Verification items for the finished model (mm, model axes). A direction names the side the tool comes from. Give positions to 0.01 mm unless a question says otherwise; leave off trailing zeros. Write each loop counter-clockwise with the first axis right and the second up, starting at its lowest first coordinate (ties: lowest second). Pieces come first, ordered by that corner, then holes. Notation, with made-up numbers: M -27.75,71.5 L 12.25,71.5 A25 cw 12.25,92.5 Z; hole C 0,80 d8. An arc over 180 degrees is marked long. Answer as a JSON object with one key per item and string values.
```python
from build123d import *

# Parameters (mm, degrees)
F0_R     = 3.175
F1_DEPTH = 6.35


with BuildPart() as f1:
    # F0 (on Top) → F1 (new body)
    with BuildSketch(Plane.XY):
        with BuildLine():
            Line((39.8145, 12.7), (0, 12.7))
            Line((0, 12.7), (-39.8145, 12.7))
            Line((-39.8145, 12.7), (-39.8145, 31.75))
            Line((-39.8145, 31.75), (-62.96914, 31.75))
            ThreePointArc((-62.96914, 31.75), (-64.550414, 31.045236), (-65.083471, 29.398126))
            Line((-65.083471, 29.398126), (-65.083471, -0.106514))
            Line((-65.083471, -0.106514), (-56.196699, -29.59399))
            ThreePointArc((-56.196699, -29.59399), (-55.189961, -31.08737), (-53.51526, -31.75))
            Line((-53.51526, -31.75), (-30.2895, -31.75))
            Line((-30.2895, -31.75), (-30.2895, -12.7))
            Line((-30.2895, -12.7), (0, -12.7))
            Line((0, -12.7), (30.2895, -12.7))
            Line((30.2895, -12.7), (30.2895, -31.75))
            Line((30.2895, -31.75), (53.51526, -31.75))
            ThreePointArc((53.51526, -31.75), (55.189961, -31.08737), (56.196699, -29.59399))
            Line((56.196699, -29.59399), (65.083471, -0.106514))
            Line((65.083471, -0.106514), (65.083471, 29.398126))
            ThreePointArc((65.083471, 29.398126), (64.550414, 31.045236), (62.96914, 31.75))
            Line((62.96914, 31.75), (39.8145, 31.75))
            Line((39.8145, 31.75), (39.8145, 12.7))
        make_face()
        with Locations((46.1645, -22.225)):
            Circle(F0_R, mode=Mode.SUBTRACT)
    extrude(amount=F1_DEPTH)


solid = f1.part
```
1) Section check C-C on y = -24. Record the boundary of the cut face in (x, z).
Completed:
{"outline": "M -57.88,0 L -30.29,0 L -30.29,6.35 L -57.88,6.35 Z; M 30.29,0 L 43.53,0 L 43.53,6.35 L 30.29,6.35 Z; M 48.8,0 L 57.88,0 L 57.88,6.35 L 48.8,6.35 Z"}
2) Access from +Z, -Z, +X, -X, +Y, -Y to the whole of each face (thin tool, end or side, straight path). Record for faces 1 (the face through (30.29, -22, 3)), 2 (the face through (-1, 0, 6.35)), 3 (the face through (39.814, 22, 3)).
Completed:
{"face 1": "+Z, -Z, -Y", "face 2": "+Z, +X, -X, +Y, -Y", "face 3": "+Z, -Z, +Y"}
3) Thickness scan on L1, parallel to X at y = 23.5, z = 1; L2, parallel to X at y = -21, z = 3.25; L3, parallel to X at y = 4.5, z = 6.25. Record the ranges inside material, lowest first.
Completed:
{"L1": "x = -65.08 to -39.81, 39.81 to 65.08", "L2": "x = -58.79 to -30.29, 30.29 to 43.24, 49.09 to 58.79", "L3": "x = -65.08 to 65.08"}
4) Section check D-D on x = 36. Record the boundary of the cut face in (y, z).
Completed:
{"outline": "M -31.75,0 L 12.7,0 L 12.7,6.35 L -31.75,6.35 Z"}
5) Section check A-A on y = 23. Record the boundary of the cut face in (x, z).
Completed:
{"outline": "M -65.08,0 L -39.81,0 L -39.81,6.35 L -65.08,6.35 Z; M 39.81,0 L 65.08,0 L 65.08,6.35 L 39.81,6.35 Z"}
6) Release check for a two-part mould opening along X. For faces 4 (the face through (-65.083, 15, 3)), 5 (the face through (52, 31.75, 3)), 6 (the face through (-39.814, 22, 3)) record: pulls with the +X half, pulls with the -X half, needs draft (parallel to the pull), parting line crosses it, or undercut.
Completed:
{"face 4": "pulls with the -X half", "face 5": "needs draft", "face 6": "undercut"}
7) Go/stop test with flat-tipped pins: pin 1 (3 mm diameter, centred on x = -5.5, z = 3.5, fed in from +Y); pin 2 (1.9 mm diameter, centred on y = 15.5, z = 2, fed in from -X); pin 3 (5 mm diameter, centred on x = 46.16, y = -22.22, fed in from -Z); pin 4 (1.9 mm diameter, centred on y = -20.5, z = 1.5, fed in from +X). Record where each tip stops, or that it passes through.
Completed:
{"pin 1": "stops at y = 12.7", "pin 2": "stops at x = -65.08", "pin 3": "passes through", "pin 4": "stops at x = 59.22"}
